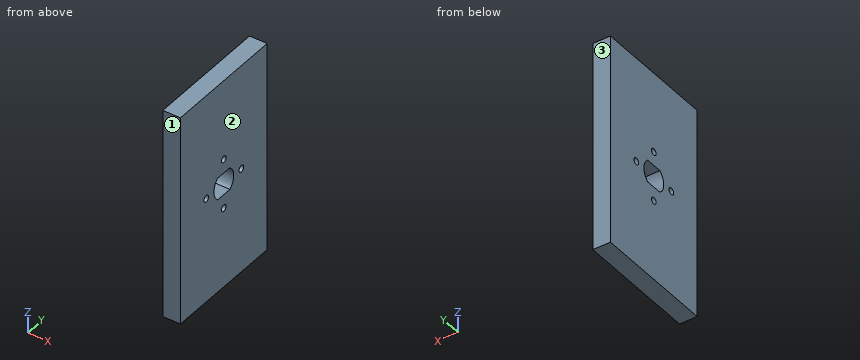
from build123d import *

# Parameters (mm, degrees)
SKETCH1_W               = 76.2
SKETCH1_H               = 44.45
BOSS_EXTRUDE1_DEPTH     = 3.175
CUT_EXTRUDE1_DEPTH      = 45.563248591
CUT_EXTRUDE1_DEPTH_BACK = 45.563248591
ADVANCEDHOLE1_START     = -3.175
ADVANCEDHOLE1_OUTLINE_R = 1.2
ADVANCEDHOLE1_DEPTH     = 6.35


# Read off the part's stored shape, not the designer's step: AdvancedHole1
with BuildPart() as part:
    # Sketch1 → Boss-Extrude1 (new, symmetric)
    with BuildSketch(Plane(origin=(0, 0, 0), x_dir=(0, 0, -1), z_dir=(1, 0, 0))):
        Rectangle(SKETCH1_W, SKETCH1_H)
    extrude(amount=BOSS_EXTRUDE1_DEPTH, both=True)

    # Sketch2 → Cut-Extrude1 (cut, two sides: drawn at the far end of the back side and taken through both)
    with BuildSketch(Plane(origin=(3.175, 0, 0), x_dir=(0, 0, -1), z_dir=(1, 0, 0)).offset(-CUT_EXTRUDE1_DEPTH_BACK)):
        with BuildLine():
            ThreePointArc((4.0005, 3.130878431), (0, 5.08), (-4.0005, 3.130878431))
            Line((-4.0005, 3.130878431), (-4.0005, -3.130878431))
            ThreePointArc((-4.0005, -3.130878431), (0, -5.08), (4.0005, -3.130878431))
            Line((4.0005, -3.130878431), (4.0005, 3.130878431))
        make_face()
    extrude(amount=CUT_EXTRUDE1_DEPTH + CUT_EXTRUDE1_DEPTH_BACK, mode=Mode.SUBTRACT)

    # AdvancedHole1 outline → AdvancedHole1 (cut)
    with BuildSketch(Plane.YZ.offset(ADVANCEDHOLE1_START)):
        with Locations((-9, 0)):
            Circle(ADVANCEDHOLE1_OUTLINE_R)
        with Locations((0, 9)):
            Circle(ADVANCEDHOLE1_OUTLINE_R)
        with Locations((9, 0)):
            Circle(ADVANCEDHOLE1_OUTLINE_R)
        with Locations((0, -9)):
            Circle(ADVANCEDHOLE1_OUTLINE_R)
    extrude(amount=ADVANCEDHOLE1_DEPTH, mode=Mode.SUBTRACT)


solid = part.part
CAD build for the part. Positions are in the model's coordinates, mm. Face numbers are marked on the shaded views. Round coordinates to 2 decimals unless told otherwise and drop trailing zeros. Order: outer loops, then holes, each group sorted by start corner. A loop starts at its lowest first (then second) coordinate and runs counter-clockwise, first axis right, second up. Notation, with made-up numbers: (23.5, 17) -> (76.5, 17) arc R27 ccw to (76.5, 56) -> close; hole circle Ø4 at (56, 83). An arc over 180 degrees is marked (long way). Write item = value, one per line. Start each with the question number.
(1) Pull direction Y, two halves, no side cores. Call the marked faces 1, 2 and 3: released by +Y, released by -Y, zero draft, split by the parting line, or undercut.
(2) Probe line 1 (Z direction, x = -0.75, y = 0); line 2 (Z direction, x = 1, y = -9); line 3 (Z direction, x = 1, y = 9.5). List the from-to ranges inside material, lowest first. Write a range as [from, to].
(3) Cut at C-C, the plane x = 1. List the corners of the cut face in (y, z) (1 decimal).
(4) Cut at A-A, the plane y = -2. List the corners of the cut face in (x, z) (1 decimal), then the cut area to 3 significant figures.
(5) Cut at D-D, the plane z = 0. List the corners of the cut face in (x, y) (3 decimals).
(6) Pin check, flat tip, straight feed: P1, Ø3, axis at y = 3, z = 0.5, coming from the +X side. Stop position of the tip, or through.
(7) Cut at B-B, the plane z = 9. List the corners of the cut face in (x, y) (3 decimals), then the cut area to 3 significant figures.
Model answer:
q1.face_1 = released by -Y
q1.face_2 = zero draft
q1.face_3 = released by +Y
q2.line_1 = [-38.1, -10.2], [-7.8, -4], [4, 7.8], [10.2, 38.1]
q2.line_2 = [-38.1, -1.2], [1.2, 38.1]
q2.line_3 = [-38.1, -1.09], [1.09, 38.1]
q3.outline = (-22.2, -38.1) -> (22.2, -38.1) -> (22.2, 38.1) -> (-22.2, 38.1) -> close; hole circle Ø2.4 at (-9, 0); hole (-3.1, -4) -> (3.1, -4) arc R5.1 ccw to (3.1, 4) -> (-3.1, 4) arc R5.1 ccw to start; hole circle Ø2.4 at (0, -9); hole circle Ø2.4 at (0, 9); hole circle Ø2.4 at (9, 0)
q4.outline = (-3.2, -38.1) -> (3.2, -38.1) -> (3.2, -4) -> (-3.2, -4) -> close; (-3.2, 4) -> (3.2, 4) -> (3.2, 38.1) -> (-3.2, 38.1) -> close
q4.area = 433 mm2
q5.outline = (-3.175, -22.225) -> (3.175, -22.225) -> (3.175, -10.2) -> (-3.175, -10.2) -> close; (-3.175, -7.8) -> (3.175, -7.8) -> (3.175, -5.08) -> (-3.175, -5.08) -> close; (-3.175, 5.08) -> (3.175, 5.08) -> (3.175, 7.8) -> (-3.175, 7.8) -> close; (-3.175, 10.2) -> (3.175, 10.2) -> (3.175, 22.225) -> (-3.175, 22.225) -> close
q6.P1 = through
q7.outline = (-3.175, -22.225) -> (3.175, -22.225) -> (3.175, -1.2) -> (-3.175, -1.2) -> close; (-3.175, 1.2) -> (3.175, 1.2) -> (3.175, 22.225) -> (-3.175, 22.225) -> close
q7.area = 267 mm2
